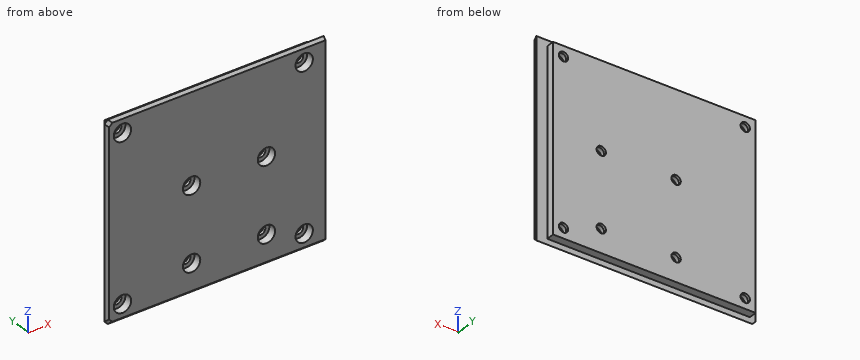
Autodesk Inventor part; units mm, degrees
ref_plane "YZ Plane" through (0, 0, 0) normal (1, 0, 0) x (0, 1, 0)
ref_plane "XZ Plane" through (0, 0, 0) normal (0, 1, 0) x (-1, 0, 0)
ref_plane "XY Plane" through (0, 0, 0) normal (0, 0, 1) x (1, 0, 0)
sketch "Sketch1" plane through (0, 0, 0) normal (0, 1, 0) x (-1, 0, 0)
  line L0 (0, 0) -> (82, 0)
  line L1 (82, 0) -> (82, -73.75)
  line L2 (82, -73.75) -> (0, -73.75)
  line L3 (0, -73.75) -> (0, 0)
  dimension "d0" = 82
  dimension "d1" = 73.75
extrude "Extrusion1" add sketch "Sketch1" along normal blind 1
sketch "Sketch2" plane through (0, 1, 0) normal (0, 1, 0) x (1, 0, 0)
  line L0 (-82, 0) -> (0, 0)
  line L1 (0, 0) -> (-4, 0)
  line L2 (-4, 0) -> (-4, 2)
  line L3 (-4, 2) -> (0, 2)
  line L4 (0, 2) -> (0, 0)
  line L5 (0, 73.75) -> (-82, 73.75)
  line L6 (0, 73.75) -> (-4, 73.75)
  line L7 (-4, 73.75) -> (-4, 71.75)
  line L8 (-4, 71.75) -> (0, 71.75)
  line L9 (0, 71.75) -> (0, 73.75)
  line L10 (0, 73.75) -> (-82, 73.75)
  line L11 (-82, 0) -> (-80, 0)
  line L12 (-80, 0) -> (-80, 2)
  line L13 (-80, 2) -> (-82, 2)
  line L14 (-82, 2) -> (-82, 0)
  line L15 (-82, 73.75) -> (-82, 0)
  line L16 (-82, 73.75) -> (-80, 73.75)
  line L17 (-80, 73.75) -> (-80, 71.75)
  line L18 (-80, 71.75) -> (-82, 71.75)
  line L19 (-82, 71.75) -> (-82, 73.75)
  line L20 (-4, 2) -> (-80, 2)
  line L21 (-80, 2) -> (-80, 71.75)
  line L22 (-80, 71.75) -> (-4, 71.75)
  line L23 (-4, 71.75) -> (-4, 2)
  dimension "d4" = 4
  dimension "d5" = 2
  dimension "d6" = 4
  dimension "d7" = 2
  dimension "d8" = 2
  dimension "d9" = 2
  dimension "d10" = 2
  dimension "d11" = 2
extrude "Extrusion2" add sketch "Sketch2" along normal blind 3 contours L21 L22 L23 L20
sketch "Sketch3" plane through (0, 0, 0) normal (0, -1, 0) x (1, 0, 0)
  line L0 (-82, -73.75) -> (-82, 0)
  line L1 (-82, -73.75) -> (-50.14, -73.75)
  line L2 (-50.14, -73.75) -> (-50.14, -62.75)
  line L3 (-50.14, -62.75) -> (-82, -62.75)
  line L4 (-82, -62.75) -> (-82, -73.75)
  line L5 (-50.14, -62.75) -> (-22.14, -62.75)
  line L6 (-22.14, -62.75) -> (-22.14, -34.75)
  line L7 (-22.14, -34.75) -> (-50.14, -34.75)
  line L8 (-50.14, -34.75) -> (-50.14, -62.75)
  circle A0 centre (-22.14, -62.75) radius 1.75
  circle A1 centre (-22.14, -34.75) radius 1.75
  circle A2 centre (-50.14, -34.75) radius 1.75
  circle A3 centre (-50.14, -62.75) radius 1.75
  point P0 (0, 0)
  point P1 (-48.39, -62.75)
  point P2 (-50.14, -61)
  point P3 (-51.89, -62.75)
  point P4 (-50.14, -64.5)
  point P5 (-23.89, -62.75)
  point P6 (-22.14, -61)
  point P7 (-22.14, -36.5)
  point P8 (-23.89, -34.75)
  point P9 (-48.39, -34.75)
  point P10 (-50.14, -36.5)
  dimension "d14" = 31.86
  dimension "d15" = 11
  dimension "d16" = 28
  dimension "d17" = 28
  dimension "d18" = 3.5
  dimension "d19" = 3.5
  dimension "d20" = 3.5
  dimension "d21" = 3.5
extrude "Extrusion3" cut sketch "Sketch3" against normal blind 5 contours A3 L8 L3 | L3 L2 A3 | L2 L5 A3 | L8 A3 L5 | A2 L7 L8 | L8 L7 A2 | A0 L6 L5 | L5 L6 A0 | A1 L6 L7 | L7 L6 A1
sketch "Sketch4" plane through (0, 0, 0) normal (0, -1, 0) x (1, 0, 0)
  circle A0 centre (-22.14, -62.75) radius 1.75
  circle A1 centre (-22.14, -62.75) radius 3.25
  circle A2 centre (-50.14, -62.75) radius 1.75
  circle A3 centre (-50.14, -62.75) radius 3.25
  circle A4 centre (-50.14, -34.75) radius 1.75
  circle A5 centre (-50.14, -34.75) radius 3.25
  circle A6 centre (-22.14, -34.75) radius 1.75
  circle A7 centre (-22.14, -34.75) radius 3.25
  point P0 (0, 0)
  dimension "d24" = 6.5
  dimension "d25" = 6.5
  dimension "d26" = 6.5
  dimension "d27" = 6.5
extrude "Extrusion4" cut sketch "Sketch4" against normal blind 3
sketch "Sketch5" plane through (0, 4, 0) normal (0, 1, 0) x (1, 0, 0)
  line L0 (-4, 71.75) -> (-80, 71.75)
  line L1 (-80, 71.75) -> (-76, 71.75)
  line L2 (-80, 71.75) -> (-76, 71.75)
  line L3 (-76, 71.75) -> (-76, 67.75)
  line L4 (-76, 67.75) -> (-80, 67.75)
  line L5 (-80, 67.75) -> (-80, 71.75)
  line L6 (-4, 71.75) -> (-8, 71.75)
  line L7 (-8, 71.75) -> (-8, 67.75)
  line L8 (-8, 67.75) -> (-4, 67.75)
  line L9 (-4, 67.75) -> (-4, 71.75)
  line L10 (-80, 2) -> (-4, 2)
  line L11 (-4, 2) -> (-8, 2)
  line L12 (-8, 2) -> (-8, 6)
  line L13 (-8, 6) -> (-4, 6)
  line L14 (-4, 6) -> (-4, 2)
  line L15 (-80, 2) -> (-76, 2)
  line L16 (-76, 2) -> (-76, 6)
  line L17 (-76, 6) -> (-80, 6)
  line L18 (-80, 6) -> (-80, 2)
  circle A0 centre (-76, 67.75) radius 1.75
  circle A1 centre (-8, 67.75) radius 1.75
  circle A2 centre (-8, 6) radius 1.75
  circle A3 centre (-76, 6) radius 1.75
  point P0 (0, 0)
  dimension "d30" = 4
  dimension "d31" = 4
  dimension "d32" = 4
  dimension "d33" = 4
  dimension "d34" = 4
  dimension "d35" = 4
  dimension "d36" = 4
  dimension "d37" = 4
  dimension "d38" = 4
  dimension "d39" = 3.5
  dimension "d40" = 3.5
  dimension "d41" = 3.5
  dimension "d42" = 3.5
extrude "Extrusion5" cut sketch "Sketch5" against normal blind 5 contours A1 L8 L7 | L7 L8 A1 | A0 L4 L3 | L3 L4 A0 | A3 L17 L16 | L16 L17 A3 | A2 L13 L12 | L12 L13 A2
sketch "Sketch6" plane through (0, 0, 0) normal (0, -1, 0) x (1, 0, 0)
  circle A0 centre (-8, -67.75) radius 1.75
  circle A1 centre (-8, -67.75) radius 3.25
  circle A2 centre (-76, -67.75) radius 1.75
  circle A3 centre (-76, -67.75) radius 3.25
  circle A4 centre (-76, -6) radius 1.75
  circle A5 centre (-76, -6) radius 3.25
  circle A6 centre (-8, -6) radius 1.75
  circle A7 centre (-8, -6) radius 3.25
  point P0 (0, 0)
  dimension "d45" = 6.5
  dimension "d46" = 6.5
  dimension "d47" = 6.5
  dimension "d48" = 6.5
extrude "Extrusion6" cut sketch "Sketch6" against normal blind 3 contours A0 | A1 | A2 | A3 | A4 | A5 | A6 | A7
sketch "Sketch7" plane through (0, 4, 0) normal (0, 1, 0) x (1, 0, 0)
  line L0 (-4, 2) -> (-4, 71.75)
  line L1 (-4, 2) -> (-4.12, 2)
  line L2 (-4.12, 2) -> (-4.12, 2.12)
  line L3 (-4.12, 2.12) -> (-4, 2.12)
  line L4 (-4, 2.12) -> (-4, 2)
  line L5 (-80, 71.75) -> (-4, 71.75)
  line L6 (-80, 71.75) -> (-79.88, 71.75)
  line L7 (-79.88, 71.75) -> (-79.88, 71.63)
  line L8 (-79.88, 71.63) -> (-80, 71.63)
  line L9 (-80, 71.63) -> (-80, 71.75)
  line L10 (-79.88, 71.63) -> (-4, 71.63)
  line L11 (-4, 71.63) -> (-4, 71.75)
  line L12 (-4, 71.75) -> (-79.88, 71.75)
  line L13 (-79.88, 71.75) -> (-79.88, 71.63)
  line L14 (-4.12, 2) -> (-4, 2)
  line L15 (-4, 2) -> (-4, 71.75)
  line L16 (-4, 71.75) -> (-4.12, 71.75)
  line L17 (-4.12, 71.75) -> (-4.12, 2)
  line L18 (-80, 2) -> (-4, 2)
  line L19 (-4.12, 2.12) -> (-80, 2.12)
  line L20 (-80, 2.12) -> (-80, 2)
  line L21 (-80, 2) -> (-4.12, 2)
  line L22 (-4.12, 2) -> (-4.12, 2.12)
  line L23 (-80, 2) -> (-79.88, 2)
  line L24 (-79.88, 2) -> (-79.88, 71.63)
  line L25 (-79.88, 71.63) -> (-80, 71.63)
  line L26 (-80, 71.63) -> (-80, 2)
  point P0 (0, 0)
  point P1 (-4.12, 2.12)
  point P2 (-79.88, 2.12)
  point P3 (-4.12, 71.63)
  dimension "d51" = 0.12
  dimension "d52" = 0.12
  dimension "d53" = 0.12
  dimension "d54" = 0.12
extrude "Extrusion7" cut sketch "Sketch7" against normal blind 3 contours L1 L2 L3 L0 | L3 L17 L10 L0 | L18 L24 L19 L2 | L10 L17 L5 L0 | L18 L20 L19 L24 | L10 L7 L5 L17 | L19 L26 L8 L24 | L8 L9 L5 L7
chamfer "Chamfer1" distance 1 angle 45 3 edges at (-41, 0, -73.75) (-82, 0, -36.875) (-41, 0, 0)
chamfer "Chamfer2" distance 1 angle 45 2 edges at (-81.5001, 0.4999, -73.2501) (-81.5001, 0.4999, -0.4999)
properties part number "Electronics Box Lid"
Geometry check sheet. Reference: the model listing, model coordinates, mm. Coordinates: 2 decimals unless noted, no trailing zeros.
Q1. Sectioned sample at A-A on z = -34.75. Give the number of separate pieces and of enclosed holes in the cut face, and give its area (3 significant figures).
Reply:
separate pieces: 3
enclosed holes: 0
area: 263 mm2
Q2. Thickness scan on probe 1 along Z at (x, y) = (-8, 2.2); probe 2 along Z at (x, y) = (-50.14, 2.4); probe 3 along X at (y, z) = (3.3, -6). Record the ranges inside material, lowest first.
Reply:
probe 1: z = -71.63 to -71, -64.5 to -9.25, -2.75 to -2.12
probe 2: z = -71.63 to -66, -59.5 to -38, -31.5 to -2.12
probe 3: x = -79.88 to -77.75, -74.25 to -9.75, -6.25 to -4.12
Q3. Depth check by flat-ended pin: pin 1 Ø4 at (x, z) = (-8, -67.75) entering from -Y; pin 2 Ø1 at (x, y) = (-66.5, 2) entering from +Z. Enter the tip coordinate at first touch or a pass-through.
Reply:
pin 1: stops at y = 3
pin 2: stops at z = -2.12
